Work out the finished part from the listing and answer in its coordinate system (mm). A direction names the side the tool comes from. Give positions to 0.01 mm unless a question says otherwise; leave off trailing zeros. Write each loop counter-clockwise with the first axis right and the second up, starting at its lowest first coordinate (ties: lowest second). Pieces come first, ordered by that corner, then holes. Notation, with made-up numbers: (64.25, 2) - (88.25, 2) arc R13 cw to (88.25, 21) - close; hole circle Ø8 at (41, 33.25). An arc over 180 degrees is marked (long way). Write item = value, one per line.
from build123d import *

# Parameters (mm, degrees)
SKETCH2_R           = 12.5
BOSS_EXTRUDE1_DEPTH = 1.5875


with BuildPart() as part:
    # Sketch2 → Boss-Extrude1 (new body, symmetric)
    with BuildSketch(Plane.XY):
        Polygon((-35, 65), (-35, 60.621778265), (-38.791651246, 62.810889132), (-43.124984579, 55.305335633), (-45.874615236, 56.892835633), (-48.874615236, 51.69668321), (-46.124984579, 50.10918321), (-54.791651246, 35.098076211), (-57.541281903, 36.685576211), (-60.541281903, 31.489423789), (-57.791651246, 29.901923789), (-66.458317913, 14.89081679), (-69.20794857, 16.47831679), (-72.20794857, 11.282164367), (-69.458317913, 9.694664367), (-73.791651246, 2.189110868), (-70, 0), (-73.791651246, -2.189110868), (-69.458317913, -9.694664367), (-72.20794857, -11.282164367), (-69.20794857, -16.47831679), (-66.458317913, -14.89081679), (-57.791651246, -29.901923789), (-60.541281903, -31.489423789), (-57.541281903, -36.685576211), (-54.791651246, -35.098076211), (-46.124984579, -50.10918321), (-48.874615236, -51.69668321), (-45.874615236, -56.892835633), (-43.124984579, -55.305335633), (-38.791651246, -62.810889132), (-35, -60.621778265), (-35, -65), (-26.333333333, -65), (-26.333333333, -68.175), (-20.333333333, -68.175), (-20.333333333, -65), (-3, -65), (-3, -68.175), (3, -68.175), (3, -65), (20.333333333, -65), (20.333333333, -68.175), (26.333333333, -68.175), (26.333333333, -65), (35, -65), (35, -60.621778265), (38.791651246, -62.810889132), (43.124984579, -55.305335633), (45.874615236, -56.892835633), (48.874615236, -51.69668321), (46.124984579, -50.10918321), (54.791651246, -35.098076211), (57.541281903, -36.685576211), (60.541281903, -31.489423789), (57.791651246, -29.901923789), (66.458317913, -14.89081679), (69.20794857, -16.47831679), (72.20794857, -11.282164367), (69.458317913, -9.694664367), (73.791651246, -2.189110868), (70, 0), (73.791651246, 2.189110868), (69.458317913, 9.694664367), (72.20794857, 11.282164367), (69.20794857, 16.47831679), (66.458317913, 14.89081679), (57.791651246, 29.901923789), (60.541281903, 31.489423789), (57.541281903, 36.685576211), (54.791651246, 35.098076211), (46.124984579, 50.10918321), (48.874615236, 51.69668321), (45.874615236, 56.892835633), (43.124984579, 55.305335633), (38.791651246, 62.810889132), (35, 60.621778265), (35, 65), (26.333333333, 65), (26.333333333, 68.175), (20.333333333, 68.175), (20.333333333, 65), (3, 65), (3, 68.175), (-3, 68.175), (-3, 65), (-20.333333333, 65), (-20.333333333, 68.175), (-26.333333333, 68.175), (-26.333333333, 65), align=None)
        Circle(SKETCH2_R, mode=Mode.SUBTRACT)
    extrude(amount=BOSS_EXTRUDE1_DEPTH, both=True)


solid = part.part
1. For a pull along X with two mould halves and no side action, classify faces 5 (the flat face through (0, 68.175, 0)), 6 (the flat face through (-70.687, 13.917, 0.022)), 7 (the flat face through (-3, -67, 0)) as pulls with the +X half, pulls with the -X half, needs draft (parallel to the pull), parting line crosses it, or undercut.
Solution:
face_5 = needs draft
face_6 = pulls with the -X half
face_7 = undercut
2. Given pin 1 (1.6 mm diameter, centred on x = 7.5, z = 0.5, fed in from -Y); pin 2 (1.6 mm diameter, centred on y = -66, z = -0.5, fed in from -X); pin 3 (1 mm diameter, centred on y = -66, z = 0, fed in from +X), each flat-ended and moving along its own axis, determine where each tip first touches the part or whether it passes through.
Solution:
pin_1 = -65
pin_2 = -26.33
pin_3 = 26.33
3. Straight lines are drawn through the part: line 1 (Y direction, x = 0, z = -0.8) (3 decimals); line 2 (Y direction, x = -57.5, z = 1.3); line 3 (Y direction, x = -27, z = 1.4). For each, find the intervals that lie inside material, in ascending order.
Solution:
line_1 = -68.175 to -12.5, 12.5 to 68.175
line_2 = -36.66 to 36.66
line_3 = -65 to 65
4. Find section A-A, the plane x = 0. Give the vertices of the cut face in (y, z) (1 decimal).
Solution:
outline = (-68.2, -1.6) - (-12.5, -1.6) - (-12.5, 1.6) - (-68.2, 1.6) - close; (12.5, -1.6) - (68.2, -1.6) - (68.2, 1.6) - (12.5, 1.6) - close
5. A tool of negligible diameter and unlimited length cuts with its end or side. For faces 1 (the flat face through (-26.333, 67, 0)), 2 (the flat face through (26.333, -67, 0)), 3 (the flat face through (-71.655, -5.889, 0.022)), 4 (the flat face through (40.93, -59.11, 0.02)), from which of +Z, -Z, +X, -X, +Y, -Y can it reach the whole face along a straight path? Write none if from no direction.
Solution:
face_1 = +Z, -Z, -X, +Y
face_2 = +Z, -Z, +X, -Y
face_3 = +Z, -Z, -X
face_4 = +Z, -Z, -Y
6. Find section B-B, the plane y = 45.5. Give the vertices of the cut face in (x, z).
Solution:
outline = (-48.79, -1.59) - (48.79, -1.59) - (48.79, 1.59) - (-48.79, 1.59) - close
